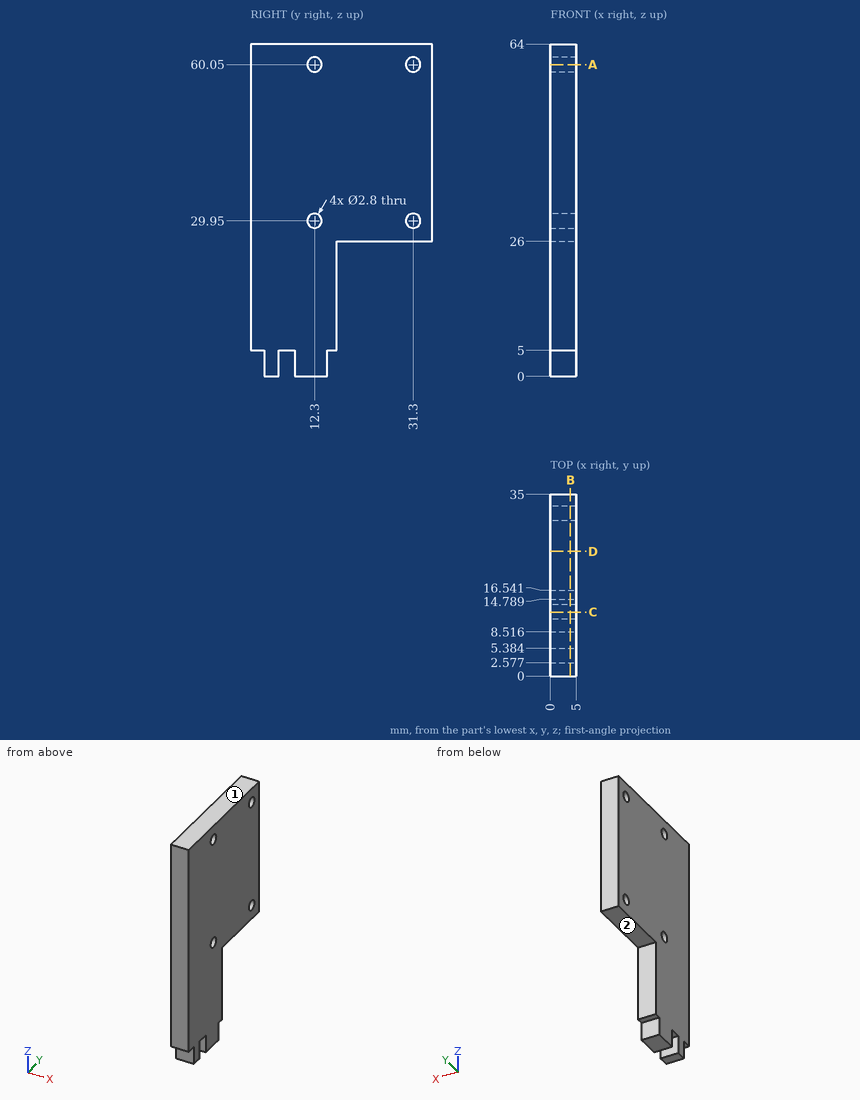
Here's the drawing with two shaded views (mm, measured from the low corner). I have some questions. A direction names the side the tool comes from. Give positions to 0.01 mm unless a question says otherwise; leave off trailing zeros. Loops run counter-clockwise (first coordinate to the right, second up) from the corner with the lowest first, then second, coordinate; pieces in that order, holes last. Notation, with made-up numbers: M 73,-40 L 92,-40 A19 ccw 92,-5 Z; hole C 8.25,17.5 d6. An arc over 180 degrees is marked long. Use one line per item in the form item = value. Start each with the question number.
(1) Please list where these lines run through material, in increasing order: line 1 (Y direction, x = 1.25, z = 60.05); line 2 (Z direction, x = 3.2, y = 31.5) (1 decimal); line 3 (Z direction, x = 4.3, y = 12).
(2) I want a section at A-A, the plane z = 60.05. Write out the boundary of the cut face in (x, y).
(3) I want a section at D-D, the plane y = 24. Write out the boundary of the cut face in (x, z).
(4) I'm going to push flat-ended pins straight in: P1, Ø1.5, axis at x = 3.5, z = 3.5, coming from the +Y side; P2, Ø1.4, axis at x = 3, y = 16, coming from the -Z side. Where does each tip first touch, or does it pass through?
(5) On a 3-axis mill with a long thin cutter (end or side, diameter ignored), from which of +Z, -Z, +X, -X, +Y, -Y can I reach the whole of each face in a straight line? I mean the marked faces 1 and 2. Say none if no direction works.
(6) I want a section at B-B, the plane x = 3.85. State how many separate pieces and enclosed holes the cut face has, and give its area (3 significant figures).
(7) I want a section at C-C, the plane y = 12.3. Write out the boundary of the cut face in (x, z), and give its area (3 significant figures).
Worked out:
q1.line_1 = 0 to 10.9, 13.7 to 29.9, 32.7 to 35
q1.line_2 = 26 to 28.6, 31.3 to 58.7, 61.4 to 64
q1.line_3 = 0 to 28.58, 31.32 to 58.68, 61.42 to 64
q2.outline = M 0,0 L 5,0 L 5,10.9 L 0,10.9 Z; M 0,13.7 L 5,13.7 L 5,29.9 L 0,29.9 Z; M 0,32.7 L 5,32.7 L 5,35 L 0,35 Z
q3.outline = M 0,26 L 5,26 L 5,64 L 0,64 Z
q4.P1 = 14.79
q4.P2 = 5
q5.face_1 = +Z, +X, -X, +Y, -Y
q5.face_2 = -Z, +X, -X, +Y
q6.separate_pieces = 1
q6.enclosed_holes = 4
q6.area = 1,700 mm²
q7.outline = M 0,0 L 5,0 L 5,28.55 L 0,28.55 Z; M 0,31.35 L 5,31.35 L 5,58.65 L 0,58.65 Z; M 0,61.45 L 5,61.45 L 5,64 L 0,64 Z
q7.area = 292 mm²
